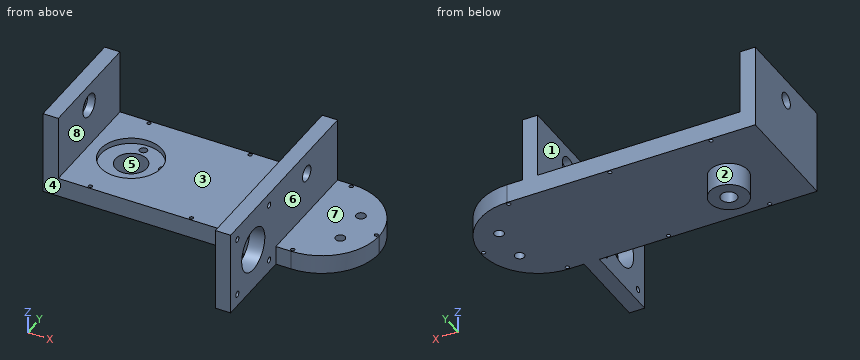
from build123d import *

# Parameters (mm, degrees)
SKETCH1_W           = 160
SKETCH1_H           = 60
BOSS_EXTRUDE1_DEPTH = 5
SKETCH4_W           = 8
SKETCH4_H           = 60
BOSS_EXTRUDE3_DEPTH = 34
CUT_EXTRUDE2_REACH  = 133.548
SKETCH5_R           = 4.1
SKETCH6_R           = 10
BOSS_EXTRUDE4_DEPTH = 12
CUT_EXTRUDE3_REACH  = 104.157
SKETCH7_R           = 4.2
LPATTERN1_COUNT     = 2
LPATTERN1_PITCH     = 114
CUT_EXTRUDE4_REACH  = 183.218
SKETCH8_R           = 4.1
CUT_EXTRUDE5_REACH  = 93.957
SKETCH9_R           = 2.5
FILLET1_R           = 30
CUT_EXTRUDE7_REACH  = 93.957
SKETCH12_R          = 1
SKETCH15_R          = 16
CUT_EXTRUDE11_DEPTH = 3
SKETCH16_R          = 8.2
CUT_EXTRUDE12_DEPTH = 12
SKETCH17_R          = 2
CUT_EXTRUDE13_DEPTH = 3
SKETCH18_W          = 8
SKETCH18_H          = 44
BOSS_EXTRUDE5_DEPTH = 44
CUT_EXTRUDE15_REACH = 149.922
SKETCH20_R          = 1.5
SKETCH20_R_2        = 11.25
SKETCH21_R          = 6
CUT_EXTRUDE16_DEPTH = 4
CUT_EXTRUDE17_START = -4
SKETCH22_R          = 6
CUT_EXTRUDE17_DEPTH = 4


with BuildPart() as part:
    # Sketch1 → Boss-Extrude1 (new, symmetric)
    with BuildSketch(Plane.XY):
        Rectangle(SKETCH1_W, SKETCH1_H)
    extrude(amount=BOSS_EXTRUDE1_DEPTH, both=True)

    # Sketch4 → Boss-Extrude3 (add)
    with BuildSketch(Plane.XY.offset(5)):
        with Locations((38, 0)):
            Rectangle(SKETCH4_W, SKETCH4_H)
    boss_extrude3 = extrude(amount=BOSS_EXTRUDE3_DEPTH)

    # Sketch5 → Cut-Extrude2 (cut, up to next)
    with BuildSketch(Plane(origin=(42, 0, 0), x_dir=(0, 0, -1), z_dir=(1, 0, 0)), mode=Mode.PRIVATE) as cut_extrude2_sk1:
        with Locations(Location((-27.5, 0, 0), (0, 0, 90))):
            Circle(SKETCH5_R)
    cut_extrude2_tool1 = extrude(cut_extrude2_sk1.sketch, amount=-CUT_EXTRUDE2_REACH, mode=Mode.PRIVATE) & part.part
    add(cut_extrude2_tool1.solids().sort_by_distance((42, 0, 27.5))[0], mode=Mode.SUBTRACT)

    # Sketch6 → Boss-Extrude4 (add)
    with BuildSketch(Plane(origin=(0, 0, -5), x_dir=(-1, 0, 0), z_dir=(0, 0, -1))):
        with Locations(Location((50, 0, 0), (0, 0, 180))):
            Circle(SKETCH6_R)
    extrude(amount=BOSS_EXTRUDE4_DEPTH)

    # Sketch7 → Cut-Extrude3 (cut, up to next)
    with BuildSketch(Plane(origin=(0, 0, -17), x_dir=(-1, 0, 0), z_dir=(0, 0, -1)), mode=Mode.PRIVATE) as cut_extrude3_sk1:
        with Locations((50, 0)):
            Circle(SKETCH7_R)
    cut_extrude3_tool1 = extrude(cut_extrude3_sk1.sketch, amount=-CUT_EXTRUDE3_REACH, mode=Mode.PRIVATE) & part.part
    add(cut_extrude3_tool1.solids().sort_by_distance((-50, 0, -17))[0], mode=Mode.SUBTRACT)

    # LPattern1: Boss-Extrude3 ×2
    with Locations(*[(-i * LPATTERN1_PITCH, 0, 0) for i in range(1, LPATTERN1_COUNT)]):
        add(boss_extrude3)

    # Sketch8 → Cut-Extrude4 (cut, up to next)
    with BuildSketch(Plane(origin=(-72, 0, -55), x_dir=(0, 0, -1), z_dir=(1, 0, 0)), mode=Mode.PRIVATE) as cut_extrude4_sk1:
        with Locations(Location((-82.5, 0, 0), (0, 0, 90))):
            Circle(SKETCH8_R)
    cut_extrude4_tool1 = extrude(cut_extrude4_sk1.sketch, amount=-CUT_EXTRUDE4_REACH, mode=Mode.PRIVATE) & part.part
    add(cut_extrude4_tool1.solids().sort_by_distance((-72, 0, 27.5))[0], mode=Mode.SUBTRACT)

    # Sketch9 → Cut-Extrude5 (cut, up to next)
    with BuildSketch(Plane.XY.offset(5), mode=Mode.PRIVATE) as cut_extrude5_sk1:
        with Locations((65, 10)):
            Circle(SKETCH9_R)
    cut_extrude5_tool1 = extrude(cut_extrude5_sk1.sketch, amount=-CUT_EXTRUDE5_REACH, mode=Mode.PRIVATE) & part.part
    # Sketch9 → Cut-Extrude5 (cut, up to next)
    with BuildSketch(Plane.XY.offset(5), mode=Mode.PRIVATE) as cut_extrude5_sk2:
        with Locations((65, -10)):
            Circle(SKETCH9_R)
    cut_extrude5_tool2 = extrude(cut_extrude5_sk2.sketch, amount=-CUT_EXTRUDE5_REACH, mode=Mode.PRIVATE) & part.part
    add(cut_extrude5_tool1.solids().sort_by_distance((65, 10, 5))[0], mode=Mode.SUBTRACT)
    add(cut_extrude5_tool2.solids().sort_by_distance((65, -10, 5))[0], mode=Mode.SUBTRACT)

    # Fillet1
    fillet1_edges = [part.edges().sort_by_distance(p)[0] for p in [
        (80, 30, 0),
        (80, -30, 0),
    ]]
    fillet(fillet1_edges, radius=FILLET1_R - 0.0001)  # a hair under: the kernel refuses the full size

    # Sketch12 → Cut-Extrude7 (cut, up to next)
    with BuildSketch(Plane.XY.offset(5), mode=Mode.PRIVATE) as cut_extrude7_sk1:
        with Locations((-3, 28.5)):
            Circle(SKETCH12_R)
    cut_extrude7_tool1 = extrude(cut_extrude7_sk1.sketch, amount=-CUT_EXTRUDE7_REACH, mode=Mode.PRIVATE) & part.part
    # Sketch12 → Cut-Extrude7 (cut, up to next)
    with BuildSketch(Plane.XY.offset(5), mode=Mode.PRIVATE) as cut_extrude7_sk2:
        with Locations((-56, 28.5)):
            Circle(SKETCH12_R)
    cut_extrude7_tool2 = extrude(cut_extrude7_sk2.sketch, amount=-CUT_EXTRUDE7_REACH, mode=Mode.PRIVATE) & part.part
    # Sketch12 → Cut-Extrude7 (cut, up to next)
    with BuildSketch(Plane.XY.offset(5), mode=Mode.PRIVATE) as cut_extrude7_sk3:
        with Locations((78.5, 0)):
            Circle(SKETCH12_R)
    cut_extrude7_tool3 = extrude(cut_extrude7_sk3.sketch, amount=-CUT_EXTRUDE7_REACH, mode=Mode.PRIVATE) & part.part
    # Sketch12 → Cut-Extrude7 (cut, up to next)
    with BuildSketch(Plane.XY.offset(5), mode=Mode.PRIVATE) as cut_extrude7_sk4:
        with Locations((50, 28.5)):
            Circle(SKETCH12_R)
    cut_extrude7_tool4 = extrude(cut_extrude7_sk4.sketch, amount=-CUT_EXTRUDE7_REACH, mode=Mode.PRIVATE) & part.part
    # Sketch12 → Cut-Extrude7 (cut, up to next)
    with BuildSketch(Plane.XY.offset(5), mode=Mode.PRIVATE) as cut_extrude7_sk5:
        with Locations((-3, -28.5)):
            Circle(SKETCH12_R)
    cut_extrude7_tool5 = extrude(cut_extrude7_sk5.sketch, amount=-CUT_EXTRUDE7_REACH, mode=Mode.PRIVATE) & part.part
    # Sketch12 → Cut-Extrude7 (cut, up to next)
    with BuildSketch(Plane.XY.offset(5), mode=Mode.PRIVATE) as cut_extrude7_sk6:
        with Locations((-56, -28.5)):
            Circle(SKETCH12_R)
    cut_extrude7_tool6 = extrude(cut_extrude7_sk6.sketch, amount=-CUT_EXTRUDE7_REACH, mode=Mode.PRIVATE) & part.part
    # Sketch12 → Cut-Extrude7 (cut, up to next)
    with BuildSketch(Plane.XY.offset(5), mode=Mode.PRIVATE) as cut_extrude7_sk7:
        with Locations((50, -28.5)):
            Circle(SKETCH12_R)
    cut_extrude7_tool7 = extrude(cut_extrude7_sk7.sketch, amount=-CUT_EXTRUDE7_REACH, mode=Mode.PRIVATE) & part.part
    add(cut_extrude7_tool1.solids().sort_by_distance((-3, 28.5, 5))[0], mode=Mode.SUBTRACT)
    add(cut_extrude7_tool2.solids().sort_by_distance((-56, 28.5, 5))[0], mode=Mode.SUBTRACT)
    add(cut_extrude7_tool3.solids().sort_by_distance((78.5, 0, 5))[0], mode=Mode.SUBTRACT)
    add(cut_extrude7_tool4.solids().sort_by_distance((50, 28.5, 5))[0], mode=Mode.SUBTRACT)
    add(cut_extrude7_tool5.solids().sort_by_distance((-3, -28.5, 5))[0], mode=Mode.SUBTRACT)
    add(cut_extrude7_tool6.solids().sort_by_distance((-56, -28.5, 5))[0], mode=Mode.SUBTRACT)
    add(cut_extrude7_tool7.solids().sort_by_distance((50, -28.5, 5))[0], mode=Mode.SUBTRACT)

    # Sketch15 → Cut-Extrude11 (cut)
    with BuildSketch(Plane.XY.offset(5)):
        with Locations((-50, 0)):
            Circle(SKETCH15_R)
    extrude(amount=-CUT_EXTRUDE11_DEPTH, mode=Mode.SUBTRACT)

    # Sketch16 → Cut-Extrude12 (cut)
    with BuildSketch(Plane.XY.offset(2)):
        with Locations((-50, 0)):
            Circle(SKETCH16_R)
    extrude(amount=-CUT_EXTRUDE12_DEPTH, mode=Mode.SUBTRACT)

    # Sketch17 → Cut-Extrude13 (cut)
    with BuildSketch(Plane.XY.offset(2)):
        with Locations((-50, 12)):
            Circle(SKETCH17_R)
        with Locations((-38, 15)):
            Circle(SKETCH17_R)
        with Locations((-35, 3)):
            Circle(SKETCH17_R)
        with Locations((-47, 0)):
            Circle(SKETCH17_R)
    extrude(amount=-CUT_EXTRUDE13_DEPTH, mode=Mode.SUBTRACT)

    # Sketch18 → Boss-Extrude5 (add)
    with BuildSketch(Plane(origin=(0, -30, 0), x_dir=(1, 0, 0), z_dir=(0, 1, 0))):
        with Locations((38, -17)):
            Rectangle(SKETCH18_W, SKETCH18_H)
    extrude(amount=-BOSS_EXTRUDE5_DEPTH)

    # Sketch20 → Cut-Extrude15 (cut, up to next)
    with BuildSketch(Plane(origin=(42, 0, 0), x_dir=(0, 0, -1), z_dir=(1, 0, 0)), mode=Mode.PRIVATE) as cut_extrude15_sk1:
        with Locations((-32.5, -36.5)):
            Circle(SKETCH20_R)
    cut_extrude15_tool1 = extrude(cut_extrude15_sk1.sketch, amount=-CUT_EXTRUDE15_REACH, mode=Mode.PRIVATE) & part.part
    # Sketch20 → Cut-Extrude15 (cut, up to next)
    with BuildSketch(Plane(origin=(42, 0, 0), x_dir=(0, 0, -1), z_dir=(1, 0, 0)), mode=Mode.PRIVATE) as cut_extrude15_sk2:
        with Locations((-1.5, -36.5)):
            Circle(SKETCH20_R)
    cut_extrude15_tool2 = extrude(cut_extrude15_sk2.sketch, amount=-CUT_EXTRUDE15_REACH, mode=Mode.PRIVATE) & part.part
    # Sketch20 → Cut-Extrude15 (cut, up to next)
    with BuildSketch(Plane(origin=(42, 0, 0), x_dir=(0, 0, -1), z_dir=(1, 0, 0)), mode=Mode.PRIVATE) as cut_extrude15_sk3:
        with Locations((-1.5, -67.5)):
            Circle(SKETCH20_R)
    cut_extrude15_tool3 = extrude(cut_extrude15_sk3.sketch, amount=-CUT_EXTRUDE15_REACH, mode=Mode.PRIVATE) & part.part
    # Sketch20 → Cut-Extrude15 (cut, up to next)
    with BuildSketch(Plane(origin=(42, 0, 0), x_dir=(0, 0, -1), z_dir=(1, 0, 0)), mode=Mode.PRIVATE) as cut_extrude15_sk4:
        with Locations((-32.5, -67.5)):
            Circle(SKETCH20_R)
    cut_extrude15_tool4 = extrude(cut_extrude15_sk4.sketch, amount=-CUT_EXTRUDE15_REACH, mode=Mode.PRIVATE) & part.part
    # Sketch20 → Cut-Extrude15 (cut, up to next)
    with BuildSketch(Plane(origin=(42, 0, 0), x_dir=(0, 0, -1), z_dir=(1, 0, 0)), mode=Mode.PRIVATE) as cut_extrude15_sk5:
        with Locations((-17, -52)):
            Circle(SKETCH20_R_2)
    cut_extrude15_tool5 = extrude(cut_extrude15_sk5.sketch, amount=-CUT_EXTRUDE15_REACH, mode=Mode.PRIVATE) & part.part
    add(cut_extrude15_tool1.solids().sort_by_distance((42, -36.5, 32.5))[0], mode=Mode.SUBTRACT)
    add(cut_extrude15_tool2.solids().sort_by_distance((42, -36.5, 1.5))[0], mode=Mode.SUBTRACT)
    add(cut_extrude15_tool3.solids().sort_by_distance((42, -67.5, 1.5))[0], mode=Mode.SUBTRACT)
    add(cut_extrude15_tool4.solids().sort_by_distance((42, -67.5, 32.5))[0], mode=Mode.SUBTRACT)
    add(cut_extrude15_tool5.solids().sort_by_distance((42, -52, 17))[0], mode=Mode.SUBTRACT)

    # Sketch21 → Cut-Extrude16 (cut)
    with BuildSketch(Plane(origin=(-72, 0, 0), x_dir=(0, 0, -1), z_dir=(1, 0, 0))):
        with Locations((-27.5, 0)):
            Circle(SKETCH21_R)
    extrude(amount=-CUT_EXTRUDE16_DEPTH, mode=Mode.SUBTRACT)

    # Sketch22 → Cut-Extrude17 (cut)
    with BuildSketch(Plane.ZY.offset(-34).offset(CUT_EXTRUDE17_START)):
        with Locations(Location((27.5, 0, 0), (0, 0, 180))):
            Circle(SKETCH22_R)
    extrude(amount=CUT_EXTRUDE17_DEPTH, mode=Mode.SUBTRACT)


solid = part.part
Geometry: final body of the model. Coordinates: model frame, mm. Face numbers are marked on the shaded views. A direction names the side the tool comes from. Round coordinates to 2 decimals unless told otherwise and drop trailing zeros. Order: outer loops, then holes, each group sorted by start corner. A loop starts at its lowest first (then second) coordinate and runs counter-clockwise, first axis right, second up.
Q1. Section C-C, the plane x = -69. Output: boundary loops of the cut face in (y, z), and give its area (3 significant figures).
Result sheet:
outline: (-30, -5) - (30, -5) - (30, 5) - (-30, 5) - close
area: 600 mm2
Q2. Section A-A, the plane z = 17. Output: boundary loops of the cut face in (x, y), and give its area (3 significant figures).
Result sheet:
outline: (-80, -30) - (-72, -30) - (-72, 30) - (-80, 30) - close; (34, -74) - (42, -74) - (42, -63.25) - (34, -63.25) - close; (34, -40.75) - (42, -40.75) - (42, 30) - (34, 30) - close
area: 1,130 mm2
Q3. Mould query, pull axis X, two halves, no side actions, for the marked faces 6, 7 and 8. Classes: released by +X, released by -X, zero draft, split by the parting line, or undercut.
Result sheet:
face 6: released by +X
face 7: zero draft
face 8: undercut
Q4. Material intervals for probe 1 along Y at (x, z) = (50, 2); probe 2 along Y at (x, z) = (-50, -1.25); probe 3 along X at (y, z) = (23.5, 25), sorted ascending.
Result sheet:
probe 1: y = -30 to -29.5, -27.5 to 27.5, 29.5 to 30
probe 2: y = -30 to -8.2, 8.2 to 30
probe 3: x = -80 to -72, 34 to 42
Q5. Access query for the marked faces 1, 2, 3, 4 and 5. Directions: +Z, -Z, +X, -X, +Y, -Y. A direction counts if a zero-diameter tool reaches every point of the face in a straight line with its end or side. Return the directions, or none.
Result sheet:
face 1: +Z, -Y
face 2: -Z
face 3: +Z, +Y, -Y
face 4: +Z, -Z, -X, -Y
face 5: +Z
Q6. Pin query (flat end, axial travel): pin 1 (4.5 mm diameter, centred on x = -34, y = 3, fed in from +Z); pin 2 (8 mm diameter, centred on x = 44.5, y = 10, fed in from -Z); pin 3 (5 mm diameter, centred on y = -67.5, z = 32.5, fed in from +X); pin 4 (12 mm diameter, centred on x = 25, z = 24.5, fed in from +Y). Return the tip coordinate at first contact, or that it passes through.
Result sheet:
pin 1: stops at z = 5
pin 2: stops at z = -5
pin 3: stops at x = 42
pin 4: passes through
Q7. Section B-B, the plane y = -54.5. Output: boundary loops of the cut face in (x, z).
Result sheet:
outline: (34, -5) - (42, -5) - (42, 6.03) - (34, 6.03) - close; (34, 27.97) - (42, 27.97) - (42, 39) - (34, 39) - close
Q8. Section D-D, the plane y = -24.5. Output: boundary loops of the cut face in (x, z).
Result sheet:
outline: (-80, -5) - (67.31, -5) - (67.31, 5) - (42, 5) - (42, 39) - (34, 39) - (34, 5) - (-72, 5) - (-72, 39) - (-80, 39) - close
